For this review, take the finished solid that the model builds, in its own axes (mm). A direction names the side the tool comes from. Give positions to 0.01 mm unless a question says otherwise; leave off trailing zeros. Loops run counter-clockwise (first coordinate to the right, second up) from the corner with the lowest first, then second, coordinate; pieces in that order, holes last. Notation, with made-up numbers: (50, 27.5) -> (95, 27.5) arc R23 cw to (95, 65.5) -> close; hole circle Ø1 at (16, 51.5). An arc over 180 degrees is marked (long way). One line per question, with ' | ' between items. Start each with the question number.
(1) Consider section B-B (z = 0). Write out the cut boundary in (x, y).
(2) Wall thickness on probe 1 along Z at (x, y) = (0, -19.25); probe 2 along X at (y, z) = (-12.5, -20.5); probe 3 along Z at (x, y) = (20, -2): over which ranges is each line inside the solid? List them lowest first.
(3) Consider section A-A (x = 0). Write out the cut boundary in (y, z).
(4) Insertion check: P1, Ø3, axis at x = 7, y = -15, coming from the +Z side; P2, Ø6, axis at x = 2, z = -11.5, coming from the +Y side; P3, Ø5, axis at x = -15, y = -16, coming from the +Z side; P4, Ø8, axis at y = -12.5, z = -11.5, coming from the +X side. Each pin has a flat end and moves straight along its axis. Give the tip position at first contact, or say it passes through.
(5) Draft analysis for pull direction X (two halves, no side actions). For faces 1 (the flat face through (-27.644, -12.325, 11.481)), 2 (the flat face through (21.146, -12.325, -17.62)), 3 (the flat face through (-8, -12, -26)), state which applies: +X half, -X half, draft (parallel to the pull), parting line (faces both ways), or undercut.
(6) Consider section D-D (y = -21.75). Give the number of separate pieces and of enclosed holes in the cut face, and give its area (3 significant figures).
(7) Consider section C-C (x = -14.5). Write out the cut boundary in (y, z), and give its area (3 significant figures).
(8) Tool access review of faces 4 (the cylindrical face through (24.514, -12.325, -4.903)), 5 (the flat face through (2.493, -12.325, -27.412)), 6 (the flat face through (-2.493, -12.325, 27.412)): name each direction out of +Z, -Z, +X, -X, +Y, -Y from which nothing blocks a thin tool from reaching the whole face with its end or side.
from build123d import *

# Parameters (mm, degrees)
F0_R     = 3
F0_R_2   = 7.5
F1_DEPTH = 25


with BuildPart() as f1:
    # F0 (on Front) → F1 (new body)
    with BuildSketch(Plane.XZ):
        with BuildLine():
            ThreePointArc((24.819347, -3), (24.954796, -1.502717), (25, 0))
            ThreePointArc((25, 0), (24.954796, 1.502717), (24.819347, 3))
            ThreePointArc((24.819347, 3), (24.519632, 4.877258), (24.078137, 6.726314))
            ThreePointArc((24.078137, 6.726314), (23.096988, 9.567086), (21.782037, 12.269592))
            ThreePointArc((21.782037, 12.269592), (20.78674, 13.889256), (19.671249, 15.428608))
            ThreePointArc((19.671249, 15.428608), (17.67767, 17.67767), (15.428608, 19.671249))
            ThreePointArc((15.428608, 19.671249), (13.889256, 20.78674), (12.269592, 21.782037))
            ThreePointArc((12.269592, 21.782037), (9.567086, 23.096988), (6.726314, 24.078137))
            ThreePointArc((6.726314, 24.078137), (4.877258, 24.519632), (3, 24.819347))
            ThreePointArc((3, 24.819347), (0, 25), (-3, 24.819347))
            ThreePointArc((-3, 24.819347), (-4.877258, 24.519632), (-6.726314, 24.078137))
            ThreePointArc((-6.726314, 24.078137), (-9.567086, 23.096988), (-12.269592, 21.782037))
            ThreePointArc((-12.269592, 21.782037), (-13.889256, 20.78674), (-15.428608, 19.671249))
            ThreePointArc((-15.428608, 19.671249), (-17.67767, 17.67767), (-19.671249, 15.428608))
            ThreePointArc((-19.671249, 15.428608), (-20.78674, 13.889256), (-21.782037, 12.269592))
            ThreePointArc((-21.782037, 12.269592), (-23.096988, 9.567086), (-24.078137, 6.726314))
            ThreePointArc((-24.078137, 6.726314), (-24.519632, 4.877258), (-24.819347, 3))
            ThreePointArc((-24.819347, 3), (-25, 0), (-24.819347, -3))
            ThreePointArc((-24.819347, -3), (-24.519632, -4.877258), (-24.078137, -6.726314))
            ThreePointArc((-24.078137, -6.726314), (-23.096988, -9.567086), (-21.782037, -12.269592))
            ThreePointArc((-21.782037, -12.269592), (-20.78674, -13.889256), (-19.671249, -15.428608))
            ThreePointArc((-19.671249, -15.428608), (-17.67767, -17.67767), (-15.428608, -19.671249))
            ThreePointArc((-15.428608, -19.671249), (-13.889256, -20.78674), (-12.269592, -21.782037))
            ThreePointArc((-12.269592, -21.782037), (-9.567086, -23.096988), (-6.726314, -24.078137))
            ThreePointArc((-6.726314, -24.078137), (-4.877258, -24.519632), (-3, -24.819347))
            ThreePointArc((-3, -24.819347), (0, -25), (3, -24.819347))
            ThreePointArc((3, -24.819347), (4.877258, -24.519632), (6.726314, -24.078137))
            ThreePointArc((6.726314, -24.078137), (9.567086, -23.096988), (12.269592, -21.782037))
            ThreePointArc((12.269592, -21.782037), (13.889256, -20.78674), (15.428608, -19.671249))
            ThreePointArc((15.428608, -19.671249), (17.67767, -17.67767), (19.671249, -15.428608))
            ThreePointArc((19.671249, -15.428608), (20.78674, -13.889256), (21.782037, -12.269592))
            ThreePointArc((21.782037, -12.269592), (23.096988, -9.567086), (24.078137, -6.726314))
            ThreePointArc((24.078137, -6.726314), (24.519632, -4.877258), (24.819347, -3))
        make_face()
        with Locations((-10.606602, -10.606602)):
            Circle(F0_R, mode=Mode.SUBTRACT)
        with Locations((5.740251, -13.858193)):
            Circle(F0_R, mode=Mode.SUBTRACT)
        with Locations((-13.858193, 5.740251)):
            Circle(F0_R, mode=Mode.SUBTRACT)
        Circle(F0_R_2, mode=Mode.SUBTRACT)
        with Locations((15, 0)):
            Circle(F0_R, mode=Mode.SUBTRACT)
        with Locations((0, 15)):
            Circle(F0_R, mode=Mode.SUBTRACT)
        with BuildLine():
            ThreePointArc((24.819347, 3), (24.954796, 1.502717), (25, 0))
            ThreePointArc((25, 0), (24.954796, -1.502717), (24.819347, -3))
            Line((24.819347, -3), (29.933259, -2))
            Line((29.933259, -2), (29.933259, 2))
            Line((29.933259, 2), (24.819347, 3))
        make_face()
        with BuildLine():
            ThreePointArc((21.782037, 12.269592), (23.096988, 9.567086), (24.078137, 6.726314))
            Line((24.078137, 6.726314), (28.420092, 9.607203))
            Line((28.420092, 9.607203), (26.889359, 13.302721))
            Line((26.889359, 13.302721), (21.782037, 12.269592))
        make_face()
        with BuildLine():
            Line((28.420092, -9.607203), (24.078137, -6.726314))
            ThreePointArc((24.078137, -6.726314), (23.096988, -9.567086), (21.782037, -12.269592))
            Line((21.782037, -12.269592), (26.889359, -13.302721))
            Line((26.889359, -13.302721), (28.420092, -9.607203))
        make_face()
        with BuildLine():
            ThreePointArc((15.428608, 19.671249), (17.67767, 17.67767), (19.671249, 15.428608))
            Line((19.671249, 15.428608), (22.580224, 19.751797))
            Line((22.580224, 19.751797), (19.751797, 22.580224))
            Line((19.751797, 22.580224), (15.428608, 19.671249))
        make_face()
        with BuildLine():
            Line((22.580224, -19.751797), (19.671249, -15.428608))
            ThreePointArc((19.671249, -15.428608), (17.67767, -17.67767), (15.428608, -19.671249))
            Line((15.428608, -19.671249), (19.751797, -22.580224))
            Line((19.751797, -22.580224), (22.580224, -19.751797))
        make_face()
        with BuildLine():
            ThreePointArc((6.726314, 24.078137), (9.567086, 23.096988), (12.269592, 21.782037))
            Line((12.269592, 21.782037), (13.302721, 26.889359))
            Line((13.302721, 26.889359), (9.607203, 28.420092))
            Line((9.607203, 28.420092), (6.726314, 24.078137))
        make_face()
        with BuildLine():
            Line((13.302721, -26.889359), (12.269592, -21.782037))
            ThreePointArc((12.269592, -21.782037), (9.567086, -23.096988), (6.726314, -24.078137))
            Line((6.726314, -24.078137), (9.607203, -28.420092))
            Line((9.607203, -28.420092), (13.302721, -26.889359))
        make_face()
        with BuildLine():
            ThreePointArc((-3, 24.819347), (0, 25), (3, 24.819347))
            Line((3, 24.819347), (2, 29.933259))
            Line((2, 29.933259), (-2, 29.933259))
            Line((-2, 29.933259), (-3, 24.819347))
        make_face()
        with BuildLine():
            Line((2, -29.933259), (3, -24.819347))
            ThreePointArc((3, -24.819347), (0, -25), (-3, -24.819347))
            Line((-3, -24.819347), (-2, -29.933259))
            Line((-2, -29.933259), (2, -29.933259))
        make_face()
        with BuildLine():
            ThreePointArc((-12.269592, 21.782037), (-9.567086, 23.096988), (-6.726314, 24.078137))
            Line((-6.726314, 24.078137), (-9.607203, 28.420092))
            Line((-9.607203, 28.420092), (-13.302721, 26.889359))
            Line((-13.302721, 26.889359), (-12.269592, 21.782037))
        make_face()
        with BuildLine():
            Line((-9.607203, -28.420092), (-6.726314, -24.078137))
            ThreePointArc((-6.726314, -24.078137), (-9.567086, -23.096988), (-12.269592, -21.782037))
            Line((-12.269592, -21.782037), (-13.302721, -26.889359))
            Line((-13.302721, -26.889359), (-9.607203, -28.420092))
        make_face()
        with BuildLine():
            ThreePointArc((-19.671249, 15.428608), (-17.67767, 17.67767), (-15.428608, 19.671249))
            Line((-15.428608, 19.671249), (-19.751797, 22.580224))
            Line((-19.751797, 22.580224), (-22.580224, 19.751797))
            Line((-22.580224, 19.751797), (-19.671249, 15.428608))
        make_face()
        with BuildLine():
            Line((-19.751797, -22.580224), (-15.428608, -19.671249))
            ThreePointArc((-15.428608, -19.671249), (-17.67767, -17.67767), (-19.671249, -15.428608))
            Line((-19.671249, -15.428608), (-22.580224, -19.751797))
            Line((-22.580224, -19.751797), (-19.751797, -22.580224))
        make_face()
        with BuildLine():
            ThreePointArc((-24.078137, 6.726314), (-23.096988, 9.567086), (-21.782037, 12.269592))
            Line((-21.782037, 12.269592), (-26.889359, 13.302721))
            Line((-26.889359, 13.302721), (-28.420092, 9.607203))
            Line((-28.420092, 9.607203), (-24.078137, 6.726314))
        make_face()
        with BuildLine():
            Line((-26.889359, -13.302721), (-21.782037, -12.269592))
            ThreePointArc((-21.782037, -12.269592), (-23.096988, -9.567086), (-24.078137, -6.726314))
            Line((-24.078137, -6.726314), (-28.420092, -9.607203))
            Line((-28.420092, -9.607203), (-26.889359, -13.302721))
        make_face()
        with BuildLine():
            ThreePointArc((-24.819347, -3), (-25, 0), (-24.819347, 3))
            Line((-24.819347, 3), (-29.933259, 2))
            Line((-29.933259, 2), (-29.933259, -2))
            Line((-29.933259, -2), (-24.819347, -3))
        make_face()
    extrude(amount=F1_DEPTH)


solid = f1.part
A:
1) outline: (-29.93, -25) -> (-7.5, -25) -> (-7.5, 0) -> (-29.93, 0) -> close; (7.5, -25) -> (12, -25) -> (12, 0) -> (7.5, 0) -> close; (18, -25) -> (29.93, -25) -> (29.93, 0) -> (18, 0) -> close
2) probe 1: z = -29.93 to -7.5, 7.5 to 12, 18 to 29.93 | probe 2: x = -21.83 to -16.66, -14.31 to 14.31, 16.66 to 21.83 | probe 3: z = -22.33 to -15.92, -15 to 15, 15.92 to 22.33
3) outline: (-25, -29.93) -> (0, -29.93) -> (0, -7.5) -> (-25, -7.5) -> close; (-25, 7.5) -> (0, 7.5) -> (0, 12) -> (-25, 12) -> close; (-25, 18) -> (0, 18) -> (0, 29.93) -> (-25, 29.93) -> close
4) P1: stops at z = 26.75 | P2: stops at y = 0 | P3: stops at z = 27.22 | P4: stops at x = 28.42
5) face 1: -X half | face 2: +X half | face 3: undercut
6) separate pieces: 1 | enclosed holes: 6 | area: 2,040 mm^2
7) outline: (-25, -20.37) -> (0, -20.37) -> (0, 2.81) -> (-25, 2.81) -> close; (-25, 8.67) -> (0, 8.67) -> (0, 20.37) -> (-25, 20.37) -> close | area: 872 mm^2
8) face 4: +X, +Y, -Y | face 5: -Z, +Y, -Y | face 6: +Z, +Y, -Y
